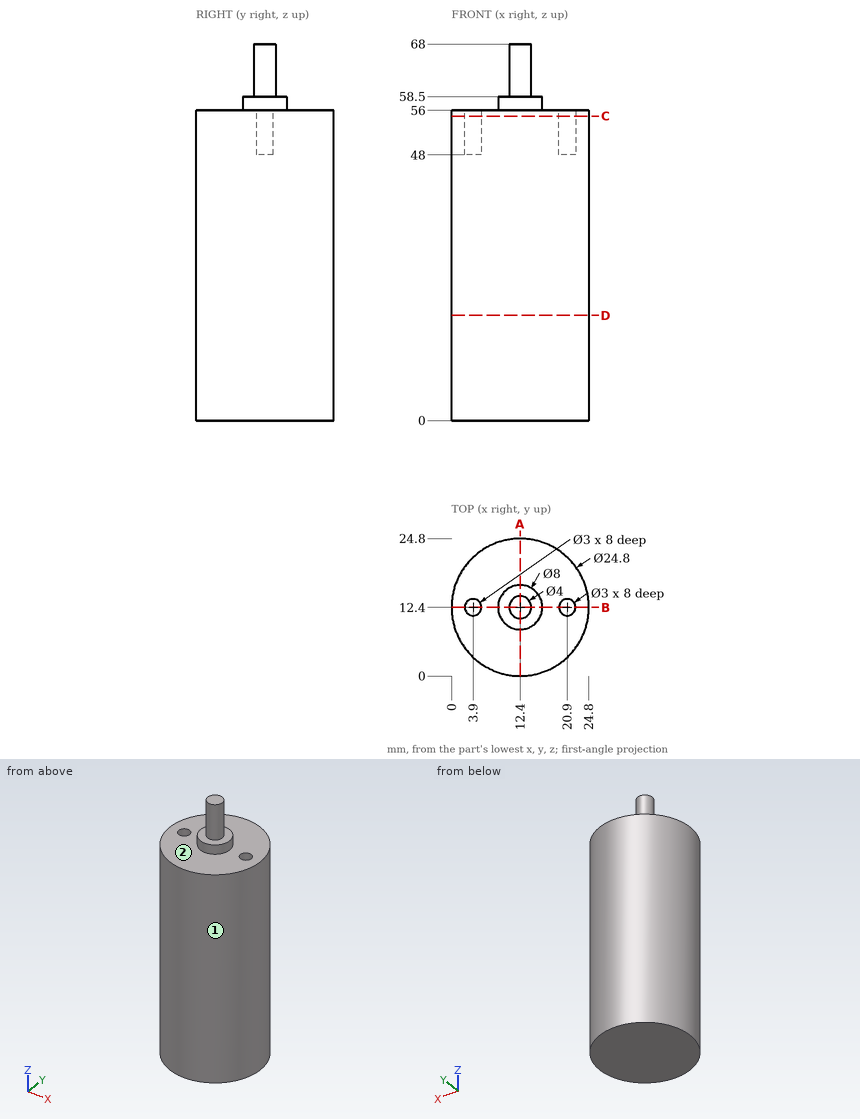
Geometry check sheet. Reference: drawing and pictorial views, mm from the part's lowest x, y, z. A direction names the side the tool comes from. Coordinates: 2 decimals unless noted, no trailing zeros. Loops run counter-clockwise (first coordinate to the right, second up) from the corner with the lowest first, then second, coordinate; pieces in that order, holes last. Notation, with made-up numbers: M -23.5,64 L 4.5,64 A17 cw 4.5,69 Z; hole C -2.75,29 d10. An arc over 180 degrees is marked long. One line per item, written item: value.
1. Section check B-B on y = 12.4. Record the cut outline in (x, z).
Answers follow:
outline: M 0,0 L 24.8,0 L 24.8,56 L 22.4,56 L 22.4,48 L 19.4,48 L 19.4,56 L 16.4,56 L 16.4,58.5 L 14.4,58.5 L 14.4,68 L 10.4,68 L 10.4,58.5 L 8.4,58.5 L 8.4,56 L 5.4,56 L 5.4,48 L 2.4,48 L 2.4,56 L 0,56 Z
2. Material ranges on line 1 along Z through (x, y) = (16.75, 12.25); line 2 along Z through (x, y) = (15.75, 12); line 3 along Y through (x, z) = (19.75, 4), recorded low to high. Write a range as from..to.
Answers follow:
line 1: 0..56
line 2: 0..58.5
line 3: 2.41..22.39
3. Section check C-C on z = 55. Record the cut outline in (x, y), plus the area to 3 significant figures.
Answers follow:
outline: C 12.4,12.4 d24.8; hole C 3.9,12.4 d3; hole C 20.9,12.4 d3
area: 469 mm^2
4. Set-up check for the marked faces 1 and 2: record each of +Z, -Z, +X, -X, +Y, -Y from which the full face is reachable in a straight line by a thin tool's end or side.
Answers follow:
face 1: +Z, -Z
face 2: +Z
5. Section check A-A on x = 12.4. Record the cut outline in (y, z).
Answers follow:
outline: M 0,0 L 24.8,0 L 24.8,56 L 16.4,56 L 16.4,58.5 L 14.4,58.5 L 14.4,68 L 10.4,68 L 10.4,58.5 L 8.4,58.5 L 8.4,56 L 0,56 Z
6. Gauge pin test, flat ends, axial feed: P1, Ø6, axis at y = 5, z = 42, coming from the +X side; P2, Ø3.5, axis at x = 3.5, y = 12.5, coming from the +Z side; P3, Ø3, axis at x = 16.5, z = 40.5, coming from the -Y side. Record the tip position at first contact, or that the pin passes through.
Answers follow:
P1: x = 23.99
P2: z = 56
P3: y = 0.28
7. Section check D-D on z = 19. Record the cut outline in (x, y).
Answers follow:
outline: C 12.4,12.4 d24.8
